The drawing under review shows one solid part. Ordinate dimensions are in mm from its lowest x, y, z. A direction names the side the tool comes from. Round coordinates to 2 decimals unless told otherwise and drop trailing zeros. Order: outer loops, then holes, each group sorted by start corner. A loop starts at its lowest first (then second) coordinate and runs counter-clockwise, first axis right, second up. Notation, with made-up numbers: M -17,36.25 L 21,36.25 A11 cw 21,45.25 Z; hole C -22,-8.5 d8. An arc over 180 degrees is marked long. Write item = value, one per line. Start each with the question number.
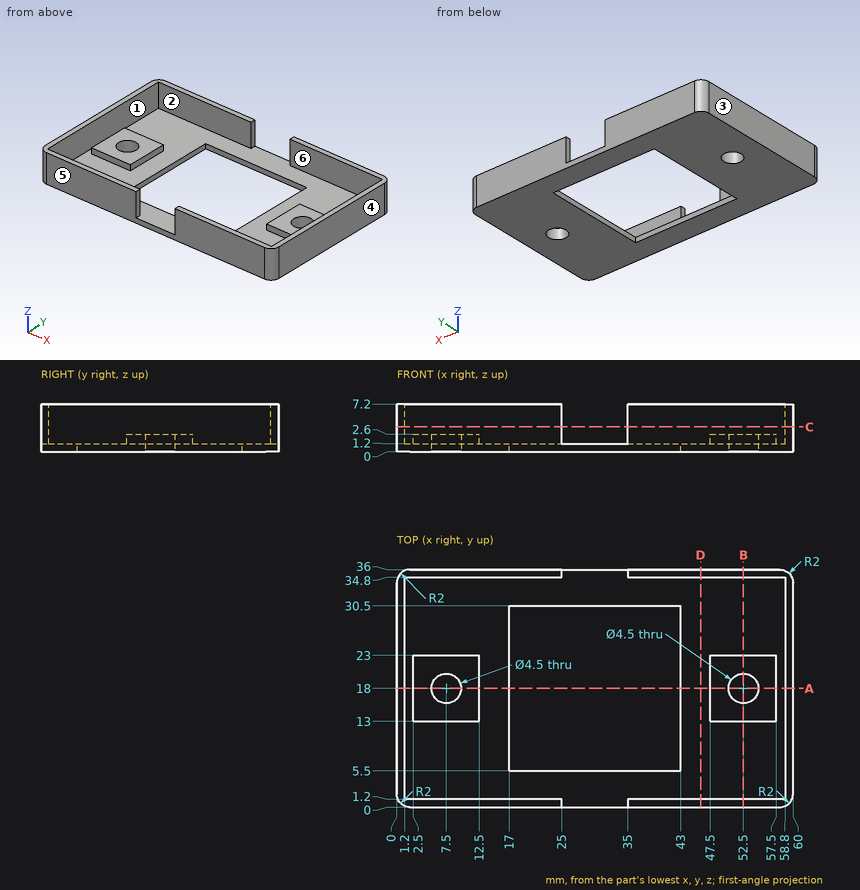
(1) Consider section C-C, the plane z = 3.75. Write out the cut boundary in (x, y).
(2) Consider section B-B, the plane x = 52.5. Write out the cut boundary in (y, z), then the cut area to 3 significant figures.
(3) Consider section A-A, the plane y = 18. Write out the cut boundary in (x, z), then the cut area to 3 significant figures.
(4) For the marked faces 5 and 6, list the 3-axis set-ups (+Z, -Z, +X, -X, +Y, -Y) from which the entire face can be reached by the end or side of a thin tool; tool diameter is ignored.
(5) Consider section D-D, the plane x = 46. Write out the cut boundary in (y, z), then the cut area to 3 significant figures.
(6) Draft analysis for pull direction X (two halves, no side actions). For the marked faces 1, 2, 3 and 4, state which applies: pulls with the +X half, pulls with the -X half, needs draft (parallel to the pull), parting line crosses it, or undercut.
(7) Insertion check: pin 1 (1 mm diameter, centred on y = 0.5, z = 4, fed in from +X); pin 2 (1.3 mm diameter, centred on y = 35.5, z = 5, fed in from -X); pin 3 (4 mm diameter, centred on x = 7.5, y = 18, fed in from -Z). Each pin has a flat end and moves straight along its axis. Give the tip position at first contact, or say it passes through.
(8) For line 1 along Y through (x, z) = (52.5, 1.65); line 2 along X through (y, z) = (4, 4.25); line 3 along Y through (x, z) = (42.5, 4.25), list the stretches that pass through material, from the lowest coordinate up. Write a range as [from, to].
Completed:
q1.outline = M 0,2 A2 ccw 2,0 L 25,0 L 25,1.2 L 1.2,1.2 L 1.2,34.8 L 25,34.8 L 25,36 L 2,36 A2 ccw 0,34 Z; M 35,0 L 58,0 A2 ccw 60,2 L 60,34 A2 ccw 58,36 L 35,36 L 35,34.8 L 58.8,34.8 L 58.8,1.2 L 35,1.2 Z
q2.outline = M 0,0 L 15.75,0 L 15.75,2.6 L 13,2.6 L 13,1.2 L 1.2,1.2 L 1.2,7.2 L 0,7.2 Z; M 20.25,0 L 36,0 L 36,7.2 L 34.8,7.2 L 34.8,1.2 L 23,1.2 L 23,2.6 L 20.25,2.6 Z
q2.area = 59.9 mm2
q3.outline = M 0,0 L 5.25,0 L 5.25,2.6 L 2.5,2.6 L 2.5,1.2 L 1.2,1.2 L 1.2,7.2 L 0,7.2 Z; M 9.75,0 L 17,0 L 17,1.2 L 12.5,1.2 L 12.5,2.6 L 9.75,2.6 Z; M 43,0 L 50.25,0 L 50.25,2.6 L 47.5,2.6 L 47.5,1.2 L 43,1.2 Z; M 54.75,0 L 60,0 L 60,7.2 L 58.8,7.2 L 58.8,1.2 L 57.5,1.2 L 57.5,2.6 L 54.75,2.6 Z
q3.area = 59.8 mm2
q4.face_5 = +Z, -Z, +X, -X, -Y
q4.face_6 = +Z
q5.outline = M 0,0 L 36,0 L 36,7.2 L 34.8,7.2 L 34.8,1.2 L 1.2,1.2 L 1.2,7.2 L 0,7.2 Z
q5.area = 57.6 mm2
q6.face_1 = undercut
q6.face_2 = undercut
q6.face_3 = pulls with the -X half
q6.face_4 = pulls with the +X half
q7.pin_1 = 59.73
q7.pin_2 = 0.19
q7.pin_3 = through
q8.line_1 = [0, 1.2], [13, 15.75], [20.25, 23], [34.8, 36]
q8.line_2 = [0, 1.2], [58.8, 60]
q8.line_3 = [0, 1.2], [34.8, 36]
